from build123d import *

# Parameters (mm, degrees)
F0_R     = 65
F1_DEPTH = 10
F3_DEPTH = 10.001
F5_R     = 62.5
F6_DEPTH = 8


with BuildPart() as f1:
    # F0 (on Front) → F1 (new body)
    with BuildSketch(Plane.XZ):
        Circle(F0_R)
    extrude(amount=F1_DEPTH)

    # F2 (on Front) → F3 (cut, through all)
    with BuildSketch(Plane.XZ):
        with BuildLine():
            Line((-104.790452, -20.48582), (-40.066584, -20.48582))
            ThreePointArc((-40.066584, -20.48582), (45, 0), (-40.066584, 20.48582))
            Line((-40.066584, 20.48582), (-167.11625, 20.48582))
            Line((-167.11625, 20.48582), (-104.790452, -20.48582))
        make_face()
    extrude(amount=F3_DEPTH, mode=Mode.SUBTRACT)

    # F5 (on offset) → F6 (cut)
    with BuildSketch(Plane.XZ.offset(1)):
        Circle(F5_R)
    extrude(amount=F6_DEPTH, mode=Mode.SUBTRACT)


solid = f1.part
Read the model definition and answer for the solid it produces. Units are mm, in the model's axes. A direction names the side the tool comes from. Coordinates: 2 decimals unless noted, no trailing zeros. Write each loop counter-clockwise with the first axis right and the second up, starting at its lowest first coordinate (ties: lowest second). Pieces come first, ordered by that corner, then holes. Notation, with made-up numbers: (-22, -13) - (16, -13) arc R25 cw to (16, 6) - close; hole circle Ø10 at (-15, 10.25). An arc over 180 degrees is marked (long way). One line per question, with ' | ' between items.
Q1. Find section B-B, the plane z = -43.5. Write down the section's boundary in (x, y), plus the area to 3 significant figures.
Result set:
outline: (-48.3, -10) - (-11.52, -10) - (-11.52, -9) - (-44.88, -9) - (-44.88, -1) - (-11.52, -1) - (-11.52, 0) - (-48.3, 0) - close; (11.52, -10) - (48.3, -10) - (48.3, 0) - (11.52, 0) - (11.52, -1) - (44.88, -1) - (44.88, -9) - (11.52, -9) - close | area: 202 mm^2
Q2. Find section C-C, the plane x = 55. Write down the section's boundary in (y, z), plus the area to 3 significant figures.
Result set:
outline: (-10, -34.64) - (0, -34.64) - (0, 34.64) - (-10, 34.64) - close; hole (-9, -29.69) - (-1, -29.69) - (-1, 29.69) - (-9, 29.69) - close | area: 218 mm^2
Q3. Consider L1, parallel to Y at x = 48.5, z = 8.5; L2, parallel to Z at x = 0, y = -5; L3, parallel to Z at x = -25, y = -5. Determine where each line is inside the solid, lowest interval first. Write a range as [from, to].
Result set:
L1: [-10, -9], [-1, 0] | L2: [-65, -62.5], [62.5, 65] | L3: [-60, -57.28], [57.28, 60]
Q4. Find section A-A, the plane x = 0. Write down the section's boundary in (y, z).
Result set:
outline: (-10, -65) - (0, -65) - (0, -45) - (-1, -45) - (-1, -62.5) - (-9, -62.5) - (-9, -45) - (-10, -45) - close; (-10, 45) - (-9, 45) - (-9, 62.5) - (-1, 62.5) - (-1, 45) - (0, 45) - (0, 65) - (-10, 65) - close
Q5. Determine the mould class of faces 4 (the cylindrical face through (64.95, -4.93, -2.57)), 5 (the flat face through (46, -9, 5)), 6 (the flat face through (43, 0, 15)) for opening direction Y: +Y half, -Y half, draft (parallel to the pull), parting line (faces both ways), or undercut.
Result set:
face 4: draft | face 5: undercut | face 6: +Y half
Q6. Find section D-D, the plane z = 52. Write down the section's boundary in (x, y), plus the area to 3 significant figures.
Result set:
outline: (-39, -10) - (39, -10) - (39, 0) - (-39, 0) - close; hole (-34.67, -9) - (34.67, -9) - (34.67, -1) - (-34.67, -1) - close | area: 225 mm^2
Q7. For faces 1 (the flat face through (-54.1, -9.4, -20.486)), 2 (the cylindrical face through (44.97, -0.49, -1.68)), 3 (the flat face through (46, -1, 5)), determine the directions among +Z, -Z, +X, -X, +Y, -Y from which every point of the face is accessible in a straight line to the end or side of a thin tool.
Result set:
face 1: -X, +Y, -Y | face 2: +Y, -Y | face 3: none
Q8. Each of these flat-tipped pins is pushed along its axis until it touches: P1, Ø4, axis at y = -8, z = 51.5, coming from the +X side; P2, Ø2, axis at y = -2.5, z = -22.5, coming from the -X side; P3, Ø3, axis at x = 18, y = -8.5, coming from the -Z side. Where does it stop, or does it pass through?
Result set:
P1: x = 42.13 | P2: x = -61.34 | P3: z = -62.87
